Read the model definition and answer for the solid it produces. Units are mm, in the model's axes. Round coordinates to 2 decimals unless told otherwise and drop trailing zeros. Order: outer loops, then holes, each group sorted by start corner. A loop starts at its lowest first (then second) coordinate and runs counter-clockwise, first axis right, second up. Notation, with made-up numbers: (29.25, 43.25) -> (55.25, 43.25) arc R10 ccw to (55.25, 60.25) -> close; hole circle Ø3 at (51, 67.25). An arc over 180 degrees is marked (long way). One line per item, written item: value. Start each with the question number.
1. A flat-ended cylindrical pin translates along its axis: pin 1 Ø5 at (x, y) = (23.97, 31.73) entering from +Z. Find the tip coordinate at first contact, or state that the pin passes through.
2. Section A-A (z = 1.75) is taken. Give the vertices of the cut face in (x, y).
3. Consider line 1 (Y direction, x = 27.5, z = 0.35); line 2 (Y direction, x = 25, z = 3.15); line 3 (Y direction, x = 7.5, z = 4.7). Determine where each line is inside the solid, lowest interval first.
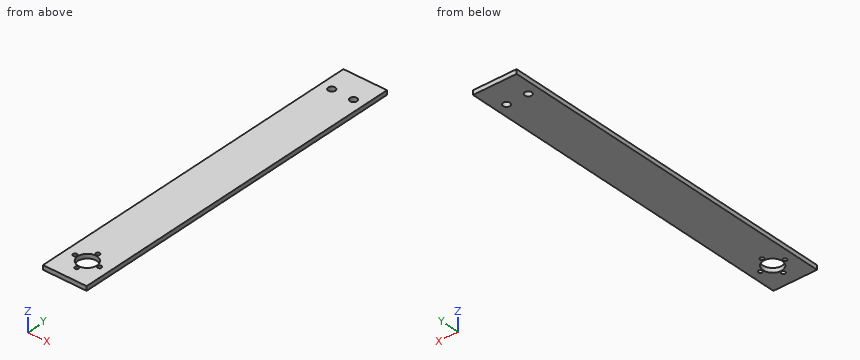
from build123d import *

# Parameters (mm, degrees)
SKETCH1_W           = 50
SKETCH1_H           = 400
SKETCH1_R           = 4
BOSS_EXTRUDE1_DEPTH = 5
SKETCH2_R           = 2.25
SKETCH2_R_2         = 11
CUT_EXTRUDE1_DEPTH  = 10


with BuildPart() as part:
    # Sketch1 → Boss-Extrude1 (new body)
    with BuildSketch(Plane.XY):
        with Locations((11.473600575, -138.26932293)):
            Rectangle(SKETCH1_W, SKETCH1_H)
        with Locations((-1.026399425, 31.73067707)):
            Circle(SKETCH1_R, mode=Mode.SUBTRACT)
        with Locations((23.973600575, 31.73067707)):
            Circle(SKETCH1_R, mode=Mode.SUBTRACT)
    extrude(amount=BOSS_EXTRUDE1_DEPTH)

    # Sketch2 → Cut-Extrude1 (cut)
    with BuildSketch(Plane(origin=(0, 0, 0), x_dir=(-1, 0, 0), z_dir=(0, 0, -1))):
        with Locations((-11.473600575, -322.39432293)):
            Circle(SKETCH2_R)
        with Locations((2.651399425, -308.26932293)):
            Circle(SKETCH2_R)
        with Locations((-11.473600575, -294.14432293)):
            Circle(SKETCH2_R)
        with Locations((-25.598600575, -308.26932293)):
            Circle(SKETCH2_R)
        with Locations((-11.473600575, -308.26932293)):
            Circle(SKETCH2_R_2)
    extrude(amount=-CUT_EXTRUDE1_DEPTH, mode=Mode.SUBTRACT)


solid = part.part
Answer:
1. pin 1: through
2. outline: (-13.53, -338.27) -> (36.47, -338.27) -> (36.47, 61.73) -> (-13.53, 61.73) -> close; hole circle Ø8 at (-1.03, 31.73); hole circle Ø4.5 at (-2.65, -308.27); hole circle Ø22 at (11.47, -308.27); hole circle Ø4.5 at (11.47, -322.39); hole circle Ø4.5 at (11.47, -294.14); hole circle Ø8 at (23.97, 31.73); hole circle Ø4.5 at (25.6, -308.27)
3. line 1: -338.27 to -309.47, -307.07 to 29.84, 33.62 to 61.73
3. line 2: -338.27 to -310.44, -306.1 to 27.86, 35.6 to 61.73
3. line 3: -338.27 to -318.53, -298.01 to 61.73
